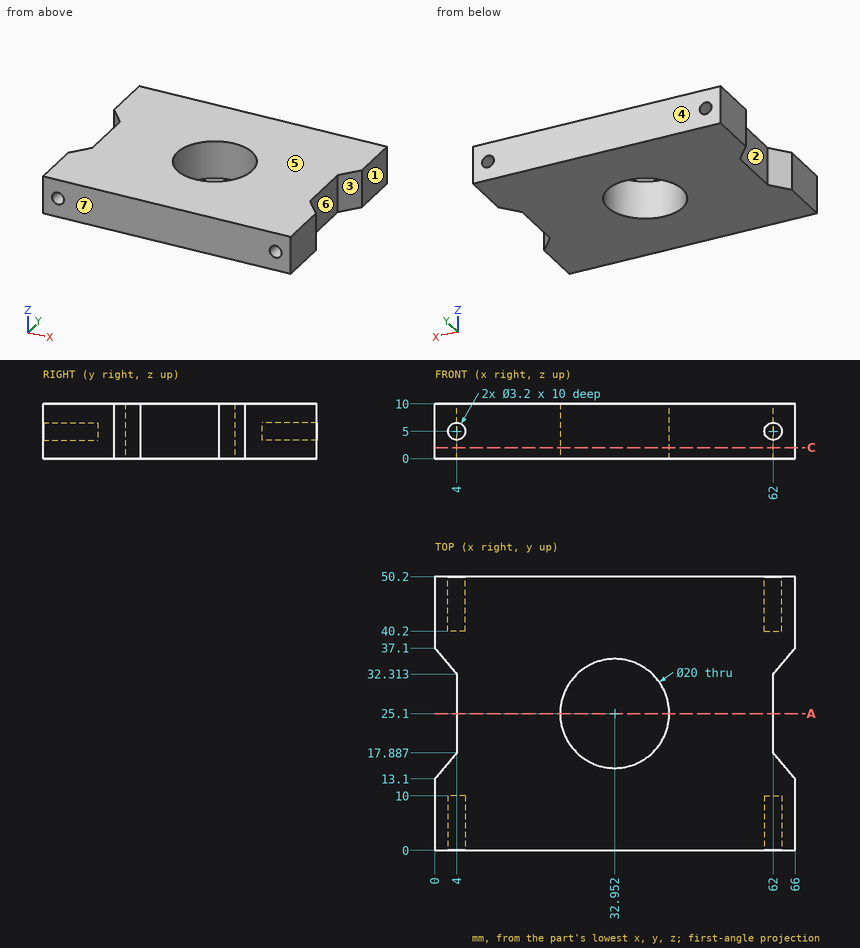
Here's the drawing with two shaded views (mm, measured from the low corner). I have some questions. A direction names the side the tool comes from. Round coordinates to 2 decimals unless told otherwise and drop trailing zeros. Loops run counter-clockwise (first coordinate to the right, second up) from the corner with the lowest first, then second, coordinate; pieces in that order, holes last. Notation, with made-up numbers: (85, 37.25) - (144, 37.25) arc R23 cw to (144, 47.25) - close; hole circle Ø2 at (31, 70.25). An arc over 180 degrees is marked (long way). Use CSV: the item, a comma, the result in double quotes. Start each with the question number.
1) If we section it at C-C on z = 2: Write out the boundary of the cut face in (x, y), plus the area to 3 significant figures.
2) We'd pull the mould along Y, two halves only. Please class the marked faces 4, 5, 6 and 7: released by +Y, released by -Y, zero draft, split by the parting line, or undercut.
3) For the marked faces 1, 2 and 3, which set-ups out of +Z, -Z, +X, -X, +Y, -Y let a thin tool reach every point of the face, with its end or its side?
4) Please list where these lines run through material, in increasing order: probe 1 along X at (y, z) = (42.5, 5); probe 2 along Z at (x, y) = (62, 5.5); probe 3 along Y at (x, z) = (32.5, 9). Write a range as [from, to].
5) If we section it at A-A on y = 25.1: Write out the boundary of the cut face in (x, z).
6) For pin 1 Ø1.6 at (x, z) = (62.5, 5.5) entering from -Y; pin 2 Ø1 at (x, z) = (4, 5) entering from +Y; pin 3 Ø6 at (y, z) = (18, 8) entering from +X; pin 4 Ø12 at (x, y) = (32.95, 25.1) entering from -Z, each with a flat end and sliding along its axis, tell me the tip position at first contact or that it passes through.
Geometry results:
1,outline,"(0, 0) - (66, 0) - (66, 13.1) - (62, 17.89) - (62, 32.31) - (66, 37.1) - (66, 50.2) - (0, 50.2) - (0, 37.1) - (4, 32.31) - (4, 17.89) - (0, 13.1) - close; hole circle Ø20 at (32.95, 25.1)"
1,area,"2,850 mm2"
2,face 4,"released by +Y"
2,face 5,"zero draft"
2,face 6,"undercut"
2,face 7,"released by -Y"
3,face 1,"+Z, -Z, +X, +Y, -Y"
3,face 2,"+Z, -Z, -X"
3,face 3,"+Z, -Z, +X"
4,probe 1,"x = [0, 2.4], [5.6, 60.4], [63.6, 66]"
4,probe 2,"z = [0, 3.4], [6.6, 10]"
4,probe 3,"y = [0, 15.11], [35.09, 50.2]"
5,outline,"(4, 0) - (22.95, 0) - (22.95, 10) - (4, 10) - close; (42.95, 0) - (62, 0) - (62, 10) - (42.95, 10) - close"
6,pin 1,"stops at y = 10"
6,pin 2,"stops at y = 40.2"
6,pin 3,"stops at x = 64.41"
6,pin 4,"passes through"
